The model under review builds one solid part; all positions refer to its coordinate system, in mm. Coordinates: 2 decimals unless noted, no trailing zeros. Order: outer loops, then holes, each group sorted by start corner. A loop starts at its lowest first (then second) coordinate and runs counter-clockwise, first axis right, second up. Notation, with made-up numbers: (63.25, 20.25) -> (99.25, 20.25) arc R26 cw to (99.25, 38.25) -> close; hole circle Ø6 at (-1, 30). An arc over 180 degrees is marked (long way). Use CSV: the item, a comma, the result in double quotes. Start each with the question number.
```python
from build123d import *

# Parameters (mm, degrees)
ESBO_O1_R                = 3.25
RESSALTO_EXTRUS_O1_DEPTH = 25
ESBO_O2_R                = 1.5
CORTE_EXTRUS_O1_DEPTH    = 26
FILETE1_R                = 0.3


with BuildPart() as part:
    # Esboço1 → Ressalto-extrusão1 (new body)
    with BuildSketch(Plane(origin=(0, 0, 0), x_dir=(1, 0, 0), z_dir=(0, 1, 0))):
        Circle(ESBO_O1_R)
    extrude(amount=RESSALTO_EXTRUS_O1_DEPTH)

    # Esboço2 → Corte-extrusão1 (cut, through all)
    with BuildSketch(Plane(origin=(0, 25, 0), x_dir=(1, 0, 0), z_dir=(0, 1, 0))):
        Circle(ESBO_O2_R)
    extrude(amount=-CORTE_EXTRUS_O1_DEPTH, mode=Mode.SUBTRACT)

    # Filete1
    filete1_edges = [part.edges().sort_by_distance(p)[0] for p in [
        (-3.25, 0, 0),
        (-3.25, 25, 0),
    ]]
    fillet(filete1_edges, radius=FILETE1_R)


solid = part.part
```
Q1. Add section B-B, the plane x = 0. State the section outline as (y, z) points.
Q2. Add section A-A, the plane z = 0. State the section outline as (x, y) points, then the cut area to 3 significant figures.
Q3. Clearance check with a flat-ended pin moving along its axis: pin 1 Ø1.5 at (x, z) = (0.5, -1) entering from -Y. State where the tip first meets the part, or that it passes through.
Q4. Draft analysis for pull direction Z (two halves, no side actions). For faces 1 (the cylindrical face through (-1.5, 12.68, -0.07)), 2 (the cylindrical face through (-2.579, 12.329, 1.978)), 3 (the flat face through (1.3, 0, 1.3)), state which applies: +Z half, -Z half, draft (parallel to the pull), parting line (faces both ways), or undercut.
Q5. To check wall thickness, follow probe 1 along X at (y, z) = (19, 0); probe 2 along Z at (x, y) = (-0.5, 19). State the ranges of each line that lie inside material, in increasing order.
Q6. Add section C-C, the plane y = 23. State the section outline as (x, z) points, then the cut area to 3 significant figures.
Answer block:
1,outline,"(0, -2.95) arc R0.3 ccw to (0.3, -3.25) -> (24.7, -3.25) arc R0.3 ccw to (25, -2.95) -> (25, -1.5) -> (0, -1.5) -> close; (0, 1.5) -> (25, 1.5) -> (25, 2.95) arc R0.3 ccw to (24.7, 3.25) -> (0.3, 3.25) arc R0.3 ccw to (0, 2.95) -> close"
2,outline,"(-3.25, 0.3) arc R0.3 ccw to (-2.95, 0) -> (-1.5, 0) -> (-1.5, 25) -> (-2.95, 25) arc R0.3 ccw to (-3.25, 24.7) -> close; (1.5, 0) -> (2.95, 0) arc R0.3 ccw to (3.25, 0.3) -> (3.25, 24.7) arc R0.3 ccw to (2.95, 25) -> (1.5, 25) -> close"
2,area,"87.4 mm²"
3,pin 1,"stops at y = 0"
4,face 1,"undercut"
4,face 2,"parting line"
4,face 3,"draft"
5,probe 1,"x = -3.25 to -1.5, 1.5 to 3.25"
5,probe 2,"z = -3.21 to -1.41, 1.41 to 3.21"
6,outline,"circle Ø6.5 at (0, 0); hole circle Ø3 at (0, 0)"
6,area,"26.1 mm²"
